Verification items for the finished model (mm, model axes). Give positions to 0.01 mm unless a question says otherwise; leave off trailing zeros. Order: outer loops, then holes, each group sorted by start corner. A loop starts at its lowest first (then second) coordinate and runs counter-clockwise, first axis right, second up.
(1) Scan lines: L1, parallel to Z at x = 0, y = 4.2; L2, parallel to Y at x = -1.25, z = 189; L3, parallel to X at y = -3.9, z = 45. Record each from-to range of solid material in increasing order.
(2) Sectioned sample at C-C on x = 0. Count the separate pieces of the cut face and the enclosed holes in it, plus the area to 3 significant figures.
(3) Sectioned sample at B-B on y = 1. Record the cut outline in (x, z).
(4) Sectioned sample at A-A on z = 298. Record the cut outline in (x, y).
```python
from build123d import *

# Parameters (mm, degrees)
SKETCH_1_W          = 9
SKETCH_1_H          = 9
EXTRUDE_1_DEPTH     = 560.3
SKETCH_2_W          = 6
SKETCH_2_H          = 6
CUT_EXTRUDE_1_DEPTH = 560.3
SKETCH_3_R          = 2.2
CUT_EXTRUDE_2_DEPTH = 582
SKETCH_4_R          = 2.2
CUT_EXTRUDE_3_DEPTH = 20


with BuildPart() as part:
    # ｽｹｯﾁ1 → ﾎﾞｽ - 押し出し1 (new body)
    with BuildSketch(Plane.XY):
        Rectangle(SKETCH_1_W, SKETCH_1_H)
    extrude(amount=EXTRUDE_1_DEPTH)

    # ｽｹｯﾁ2 → ｶｯﾄ - 押し出し1 (cut)
    with BuildSketch(Plane.XY.offset(560.3)):
        Rectangle(SKETCH_2_W, SKETCH_2_H)
    extrude(amount=-CUT_EXTRUDE_1_DEPTH, mode=Mode.SUBTRACT)

    # ｽｹｯﾁ3 → ｶｯﾄ - 押し出し2 (cut)
    with BuildSketch(Plane(origin=(0, 4.5, 0), x_dir=(1, 0, 0), z_dir=(0, 1, 0))):
        with Locations((0, -25)):
            Circle(SKETCH_3_R)
        with Locations((0, -45)):
            Circle(SKETCH_3_R)
    extrude(amount=-CUT_EXTRUDE_2_DEPTH, mode=Mode.SUBTRACT)

    # ｽｹｯﾁ4 → ｶｯﾄ - 押し出し3 (cut)
    with BuildSketch(Plane(origin=(0, 4.5, 0), x_dir=(1, 0, 0), z_dir=(0, 1, 0))):
        with Locations((0, -535.3)):
            Circle(SKETCH_4_R)
        with Locations((0, -504.3)):
            Circle(SKETCH_4_R)
    extrude(amount=-CUT_EXTRUDE_3_DEPTH, mode=Mode.SUBTRACT)


solid = part.part
```
Ans:
1. L1: z = 0 to 22.8, 27.2 to 42.8, 47.2 to 502.1, 506.5 to 533.1, 537.5 to 560.3
1. L2: y = -4.5 to -3, 3 to 4.5
1. L3: x = -4.5 to -2.2, 2.2 to 4.5
2. separate pieces: 10
2. enclosed holes: 0
2. area: 1,630 mm2
3. outline: (-4.5, 0) - (-3, 0) - (-3, 560.3) - (-4.5, 560.3) - close; (3, 0) - (4.5, 0) - (4.5, 560.3) - (3, 560.3) - close
4. outline: (-4.5, -4.5) - (4.5, -4.5) - (4.5, 4.5) - (-4.5, 4.5) - close; hole (-3, -3) - (3, -3) - (3, 3) - (-3, 3) - close
